Geometry check sheet. Reference: the model listing, model coordinates, mm. Round coordinates to 2 decimals unless told otherwise and drop trailing zeros. Loops run counter-clockwise (first coordinate to the right, second up) from the corner with the lowest first, then second, coordinate; pieces in that order, holes last. Notation, with made-up numbers: (32.25, -2.5) -> (54.25, -2.5) arc R24 ccw to (54.25, 29.5) -> close; hole circle Ø4 at (49, 52). An arc over 180 degrees is marked (long way). Use one line per item in the form item = value.
Autodesk Inventor part; units mm, degrees
ref_plane "YZ Plane" through (0, 0, 0) normal (1, 0, 0) x (0, 1, 0)
ref_plane "XZ Plane" through (0, 0, 0) normal (0, 1, 0) x (-1, 0, 0)
ref_plane "XY Plane" through (0, 0, 0) normal (0, 0, 1) x (1, 0, 0)
sketch "Sketch1" plane through (0, 0, 0) normal (0, 0, 1) x (1, 0, 0)
  circle A0 centre (1.1906, -1.1906) radius 0.3969
  arc A1 (2.3812, -1.1906) -> (0, -1.1906) centre (1.1906, -1.1906) ccw
  line L0 (1.1906, -1.1906) -> (1.1906, 0)
  line L1 (0, 0) -> (0, -18.8722)
  line L2 (0, -18.8722) -> (2.3813, -18.8722)
  line L3 (2.3813, -18.8722) -> (2.3812, -1.1906)
  circle A2 centre (1.1906, -18.8722) radius 1.5875
  point P0 (1.1906, 0)
  point P1 (0, -1.1906)
  point P2 (0, -17.8222)
  point P3 (2.3813, -17.8222)
  point P4 (2.3813, -1.1906)
  dimension "d4" = 18.8722
  dimension "d5" = 3.175
extrude "Extrusion1" add sketch "Sketch1" along normal blind 0.7937 contours L3 A2 L1 A1
properties part number "Conn Rod Rod Portion"
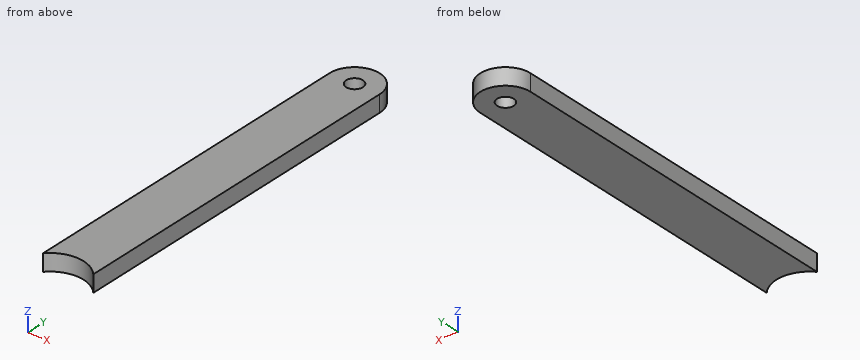
1. Section check B-B (z = 0.35). Record the boundary of the cut face in (x, y) (1 decimal), then the cut area to 3 significant figures.
Return value:
outline = (0, -17.8) arc R1.6 cw to (2.4, -17.8) -> (2.4, -1.2) arc R1.2 ccw to (0, -1.2) -> close; hole circle Ø0.8 at (1.2, -1.2)
area = 40.4 mm2
2. Section check A-A (x = 1.4). Record the boundary of the cut face in (y, z).
Return value:
outline = (-17.3, 0) -> (-1.53, 0) -> (-1.53, 0.79) -> (-17.3, 0.79) -> close; (-0.85, 0) -> (-0.02, 0) -> (-0.02, 0.79) -> (-0.85, 0.79) -> close
3. Material ranges on line 1 along Y through (x, z) = (1.4, 0.35); line 2 along Y through (x, z) = (0.25, 0.6); line 3 along Y through (x, z) = (0.3, 0.65), recorded low to high.
Return value:
line_1 = -17.3 to -1.53, -0.85 to -0.02
line_2 = -17.59 to -0.46
line_3 = -17.56 to -0.4
